Design review of the part built by this model. Coordinates are the model's own, in mm. Coordinates: 2 decimals unless noted, no trailing zeros. Order: outer loops, then holes, each group sorted by start corner. A loop starts at its lowest first (then second) coordinate and runs counter-clockwise, first axis right, second up. Notation, with made-up numbers: (58.25, 54.25) -> (112.25, 54.25) arc R19 ccw to (112.25, 70.25) -> close; hole circle Ø7 at (-8.75, 85.25). An arc over 180 degrees is marked (long way). Write item = value, one per line.
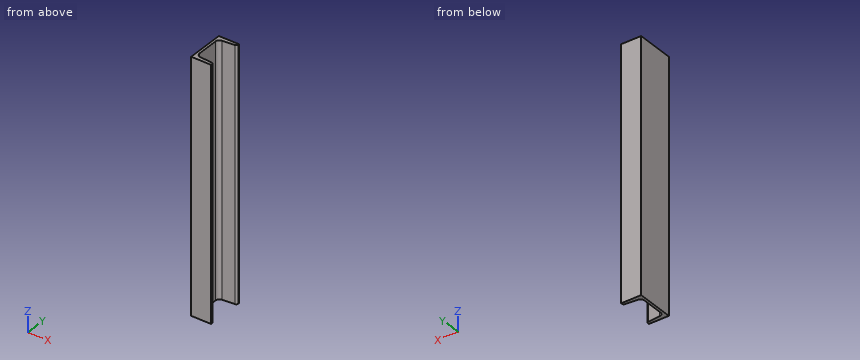
Autodesk Inventor part; units mm, degrees
ref_plane "開始平面" through (0, 0, 0) normal (0, 0, 1) x (1, 0, 0)
ref_plane "終了平面" through (0, 0, 500) normal (0, 0, 1) x (1, 0, 0)
ref_plane "YZ Plane" through (0, 0, 0) normal (1, 0, 0) x (0, 1, 0)
ref_plane "開始平面" through (0, 0, 0) normal (0, 0, 1) x (1, 0, 0)
ref_plane "終了平面" through (0, 0, 500) normal (0, 0, 1) x (1, 0, 0)
sketch "スケッチ" plane through (0, 0, 0) normal (0, 0, 1) x (1, 0, 0)
  line L0 (-12.8, 0) -> (-12.8, 37.5)
  line L1 (-12.8, 37.5) -> (27.2, 37.5)
  line L2 (27.2, 37.5) -> (27.2, 35.6964)
  line L3 (23.5486, 31.7116) -> (-0.4973, 29.6078)
  line L4 (-7.8, 21.6383) -> (-7.8, 0)
  line L5 (-7.8, 0) -> (-12.8, 0) construction
  line L6 (9.7, 37.5) -> (9.7, 30.5) construction
  line L7 (27.2, 32.0311) -> (27.2, 30.5) construction
  line L8 (27.2, 30.5) -> (9.7, 30.5) construction
  line L9 (0, 15) -> (0, -27) construction
  line L10 (-5.539, 0) -> (16.0067, 0) construction
  line L11 (-12.8, 0) -> (-12.8, -37.5)
  line L12 (-12.8, -37.5) -> (27.2, -37.5)
  line L13 (27.2, -37.5) -> (27.2, -35.6964)
  line L14 (23.5486, -31.7116) -> (-0.4973, -29.6078)
  line L15 (-7.8, -21.6383) -> (-7.8, 0)
  arc A0 (-0.4973, 29.6078) -> (-7.8, 21.6383) centre (0.2, 21.6383) ccw
  arc A1 (-7.8, -21.6383) -> (-0.4973, -29.6078) centre (0.2, -21.6383) ccw
  arc A2 (23.5486, 31.7116) -> (27.2, 35.6964) centre (23.2, 35.6964) ccw
  arc A3 (27.2, -35.6964) -> (23.5486, -31.7116) centre (23.2, -35.6964) ccw
  line L16 (0, 52.5) -> (0, -52.5) construction
  line L17 (-20.955, 0) -> (36.1298, 0) construction
  point P0 (-7.8, 28.9689)
  point P1 (27.2, -32.0311)
  point P2 (-7.8, -28.9689)
  point P3 (9.7, -37.5)
  point P4 (9.7, -30.5)
  dimension "d0" = 5
  dimension "d1" = 37.5
  dimension "d2" = 40
  dimension "d3" = 7
  dimension "d4" = 17.5
  dimension "d5" = 1.5311
  dimension "d23" = 8
  dimension "d24" = 4
  dimension "d25" = 12.8
extrude "ボディ" add sketch "スケッチ" along normal up to surface (500 mm away) from surface at 0
sketch "Sketch3" plane through (0, 0, 0) normal (0, 0, 1) x (1, 0, 0)
  line L0 (0, 0) -> (10, 0)
ref_plane "Work Plane3" through (0, 0, 0) normal (0, -1, 0) x (1, 0, 0)
sketch "Sketch4" plane through (0, 0, 0) normal (0, -1, 0) x (1, 0, 0)
  line L0 (-2, 0) -> (12, 0)
  line L1 (-2, 500) -> (12, 500)
  dimension "d29" = 500
equation "\"d0\" = G_T"
equation "\"d1\" = 0.5 * G_H"
equation "\"d2\" = G_W"
equation "\"d3\" = G_T1"
equation "\"d4\" = G_C"
equation "\"d23\" = G_IR"
equation "\"d24\" = G_ER"
equation "\"d25\" = ey"
equation "\"d6\" = G_L"
equation "\"G_W\" = 40"
equation "\"G_H\" = 75"
equation "\"G_T\" = 5"
equation "\"G_T1\" = 7"
equation "\"G_NG\" = 0.08749"
equation "\"G_ER\" = 4"
equation "\"G_IR\" = 8"
equation "\"G_C\" = 17.5"
equation "\"G_L\" = d29"
equation "\"ey\" = 12.8"
equation "\"G_OFFSET_START\" = 0"
equation "\"G_OFFSET_END\" = 0"
properties part number "JIS G 3192 - 75 x 40 x 5 - 500" material "SS400"
(1) For L1, parallel to Y at x = 0.5, z = 130.5; L2, parallel to X at y = 4, z = 286; L3, parallel to Y at x = 20.5, z = 312, list the stretches that pass through material, from the lowest coordinate up.
Report:
L1 = -37.5 to -29.7, 29.7 to 37.5
L2 = -12.8 to -7.8
L3 = -37.5 to -31.44, 31.44 to 37.5
(2) We need section A-A (x = 6.5). Write out the cut boundary in (y, z), and give its area (3 significant figures).
Report:
outline = (-37.5, 0) -> (-30.22, 0) -> (-30.22, 500) -> (-37.5, 500) -> close; (30.22, 0) -> (37.5, 0) -> (37.5, 500) -> (30.22, 500) -> close
area = 7,280 mm²
(3) Insertion check: pin 1 (12 mm diameter, centred on y = -21, z = 148, fed in from +X). The pin has a flat end and moves straight along its axis. Give the tip position at first contact, or say it passes through.
Report:
pin_1 = -5.74
(4) We need section C-C (y = -1.5). Write out the cut boundary in (x, z).
Report:
outline = (-12.8, 0) -> (-7.8, 0) -> (-7.8, 500) -> (-12.8, 500) -> close
(5) We need section B-B (z = 341). Write out the cut boundary in (x, y), and give its area (3 significant figures).
Report:
outline = (-12.8, -37.5) -> (27.2, -37.5) -> (27.2, -35.7) arc R4 ccw to (23.55, -31.71) -> (-0.5, -29.61) arc R8 cw to (-7.8, -21.64) -> (-7.8, 21.64) arc R8 cw to (-0.5, 29.61) -> (23.55, 31.71) arc R4 ccw to (27.2, 35.7) -> (27.2, 37.5) -> (-12.8, 37.5) -> close
area = 882 mm²
